Check sheet for the drawn part. Datum: minimum x, y, z corner. Units: mm. A direction names the side the tool comes from. Round coordinates to 2 decimals unless told otherwise and drop trailing zeros. Order: outer loops, then holes, each group sorted by start corner. A loop starts at its lowest first (then second) coordinate and runs counter-clockwise, first axis right, second up.
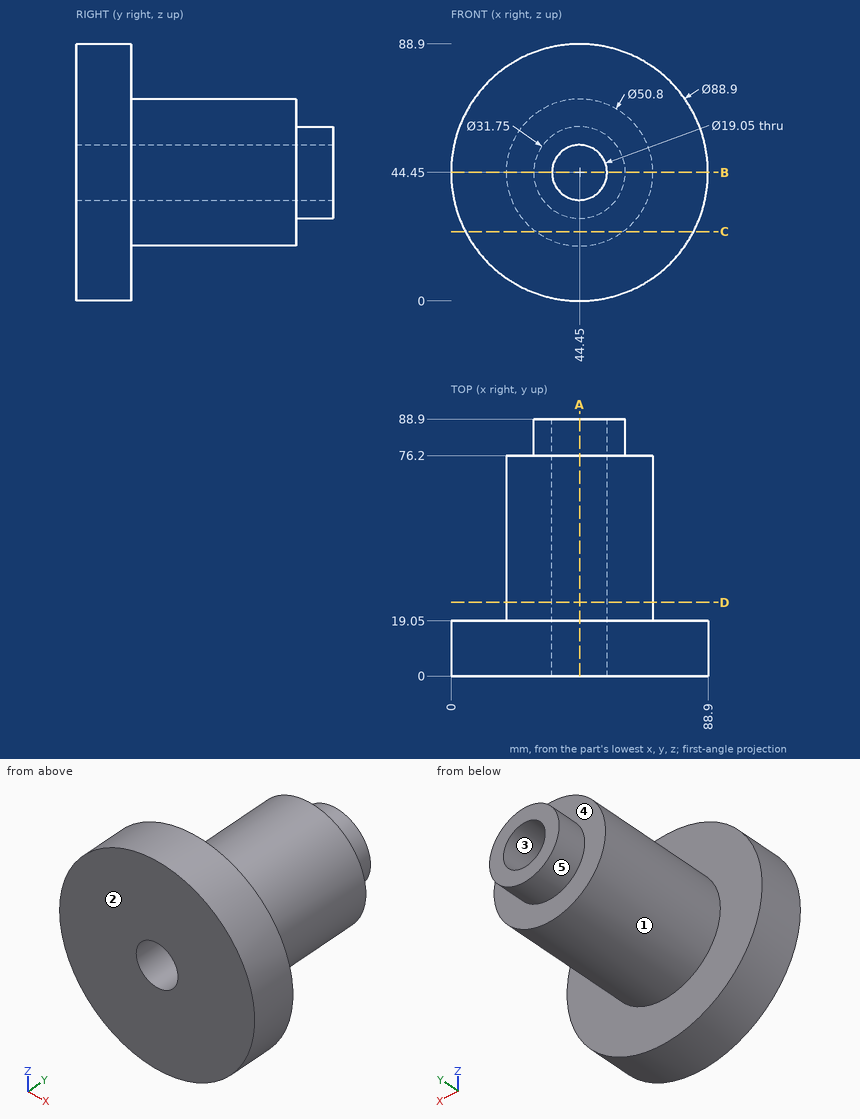
(1) Set-up check for the marked faces 1 and 2: record each of +Z, -Z, +X, -X, +Y, -Y from which the full face is reachable in a straight line by a thin tool's end or side.
Returned:
face 1: +Y
face 2: +Z, -Z, +X, -X, -Y
(2) Material ranges on line 1 (Z direction, x = 44, y = 53); line 2 (Y direction, x = 18, z = 79.5), recorded low to high.
Returned:
line 1: z = 19.05 to 34.94, 53.96 to 69.85
line 2: y = 0 to 19.05
(3) Depth check by flat-ended pin: P1, Ø4, axis at x = 61, z = 29, coming from the +Y side; P2, Ø12, axis at y = 45, z = 31, coming from the +X side; P3, Ø1, axis at x = 71.5, z = 54.5, coming from the +Y side. Enter the tip coordinate at first touch or a pass-through.
Returned:
P1: stops at y = 76.2
P2: stops at x = 68.73
P3: stops at y = 19.05
(4) Sectioned sample at A-A, the plane x = 44.45. Record the cut outline in (y, z) (3 decimals).
Returned:
outline: (0, 0) - (19.05, 0) - (19.05, 19.05) - (76.2, 19.05) - (76.2, 28.575) - (88.9, 28.575) - (88.9, 34.925) - (0, 34.925) - close; (0, 53.975) - (88.9, 53.975) - (88.9, 60.325) - (76.2, 60.325) - (76.2, 69.85) - (19.05, 69.85) - (19.05, 88.9) - (0, 88.9) - close
(5) Draft check along X on the marked faces 3, 4 and 5. Enter one of: released by +X, released by -X, zero draft, split by the parting line, or undercut.
Returned:
face 3: undercut
face 4: zero draft
face 5: split by the parting line
(6) Sectioned sample at D-D, the plane y = 25.5. Record the cut outline in (x, z) (3 decimals).
Returned:
outline: circle Ø50.8 at (44.45, 44.45); hole circle Ø19.05 at (44.45, 44.45)
(7) Sectioned sample at B-B, the plane z = 44.45. Record the cut outline in (x, y) (3 decimals), and give its area (3 significant figures).
Returned:
outline: (0, 0) - (34.925, 0) - (34.925, 88.9) - (28.575, 88.9) - (28.575, 76.2) - (19.05, 76.2) - (19.05, 19.05) - (0, 19.05) - close; (53.975, 0) - (88.9, 0) - (88.9, 19.05) - (69.85, 19.05) - (69.85, 76.2) - (60.325, 76.2) - (60.325, 88.9) - (53.975, 88.9) - close
area: 3,310 mm2
(8) Sectioned sample at C-C, the plane z = 24. Record the cut outline in (x, y), and give its area (3 significant figures).
Returned:
outline: (4.98, 0) - (83.92, 0) - (83.92, 19.05) - (59.52, 19.05) - (59.52, 76.2) - (29.38, 76.2) - (29.38, 19.05) - (4.98, 19.05) - close
area: 3,230 mm2
